Geometry check sheet. Reference: drawing and pictorial views, mm from the part's lowest x, y, z. Give positions to 0.01 mm unless a question says otherwise; leave off trailing zeros. Loops run counter-clockwise (first coordinate to the right, second up) from the corner with the lowest first, then second, coordinate; pieces in that order, holes last. Notation, with made-up numbers: (44, 24.25) - (82, 24.25) arc R3 cw to (82, 29.25) - close; hole circle Ø9 at (-33.5, 63.5). An arc over 180 degrees is marked (long way). One line per question, with ' | ' between items. Start each with the question number.
1. Thickness scan on line 1 along X through (y, z) = (6, 0.9) (1 decimal); line 2 along X through (y, z) = (51.5, 1.6) (1 decimal); line 3 along Y through (x, z) = (107, 3.15). Record the ranges inside material, lowest first. Write a range as from..to.
2. Depth check by flat-ended pin: pin 1 Ø2 at (y, z) = (29.5, 2.5) entering from -X; pin 2 Ø2 at (x, z) = (97.5, 1.5) entering from -Y. Enter the tip coordinate at first touch or a pass-through.
3. Section check B-B, the plane z = 1.7. State how many separate pieces and enclosed holes the cut face has, then the cut area to 3 significant figures.
4. Section check A-A, the plane y = 31. Enter the section's corners in (x, z) (1 decimal).
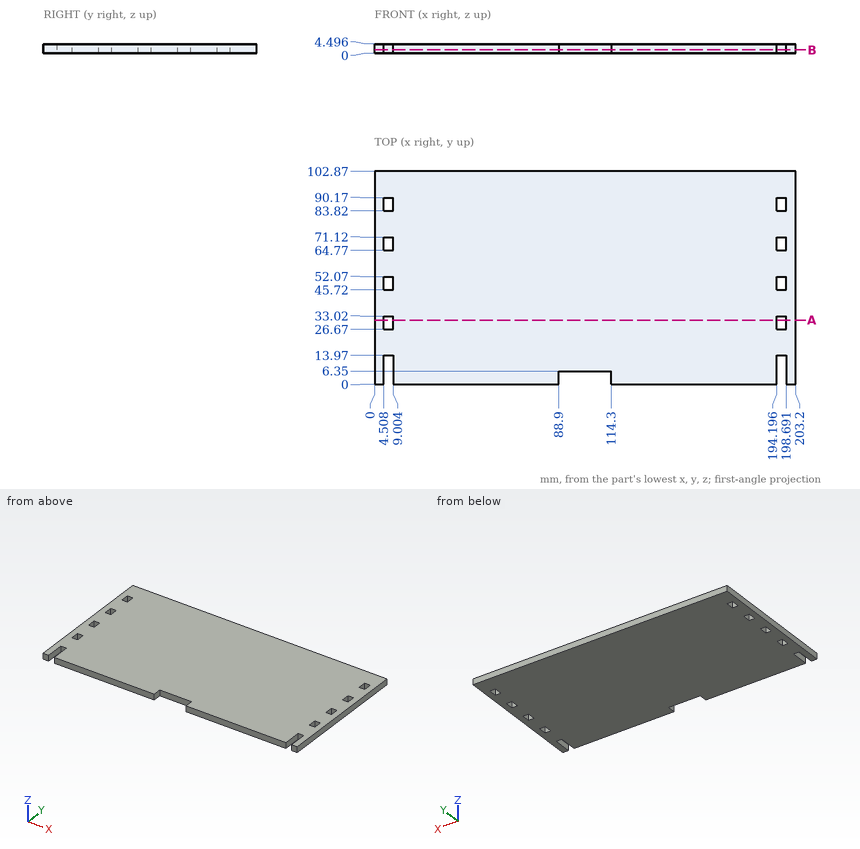
Results list:
1) line 1: 0..4.5, 9..88.9, 114.3..194.2, 198.7..203.2 | line 2: 0..4.5, 9..194.2, 198.7..203.2 | line 3: 6.35..102.87
2) pin 1: x = 0 | pin 2: y = 6.35
3) separate pieces: 1 | enclosed holes: 8 | area: 20,400 mm²
4) outline: (0, 0) - (4.5, 0) - (4.5, 4.5) - (0, 4.5) - close; (9, 0) - (194.2, 0) - (194.2, 4.5) - (9, 4.5) - close; (198.7, 0) - (203.2, 0) - (203.2, 4.5) - (198.7, 4.5) - close
